Can you work these out from the model? Positions are in its coordinate system, mm. Face numbers are marked on the shaded views. A direction names the side the tool comes from. Coordinates: 2 decimals unless noted, no trailing zeros. Write each loop counter-clockwise with the first axis right and the second up, starting at its lowest first coordinate (ties: lowest second). Pieces come first, ordered by that corner, then holes. Notation, with made-up numbers: (-8.5, -34.75) -> (21.5, -34.75) arc R17 cw to (21.5, -18.75) -> close; hole circle Ø8 at (87, 71). An arc over 180 degrees is marked (long way). Answer as CSV lines item,"result". Start each with the question number.
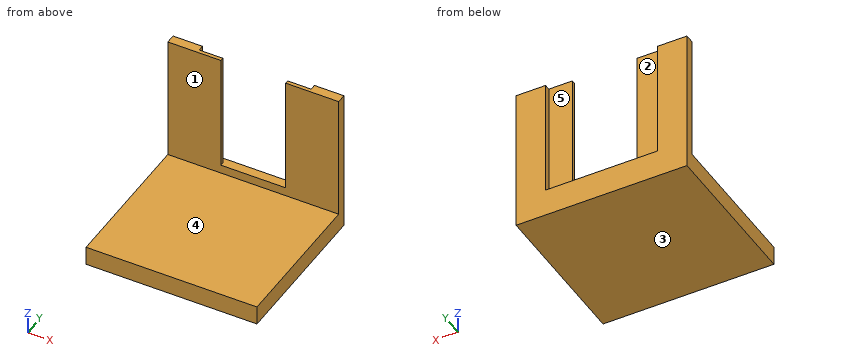
```python
from build123d import *

# Parameters (mm, degrees)
F0_W      = 38
F0_H      = 1.2
F1_DEPTH  = 20
F3_W      = 10
F3_H      = 20
F4_DEPTH  = 3.2
F5_W      = 10
F5_H      = 20
F6_DEPTH  = 3.2
F7_W      = 38
F7_H      = 2
F8_DEPTH  = 10
F2_W      = 22
F2_H      = 1.2
F9_DEPTH  = 20
F10_W     = 18
F10_H     = 7
F11_DEPTH = 50
F12_DEPTH = 20
F13_DEPTH = 40
F14_DEPTH = 0.5


with BuildPart() as f1:
    # F0 (on Top) → F1 (new body)
    with BuildSketch(Plane.XY):
        with Locations((19, 0.6)):
            Rectangle(F0_W, F0_H)
    extrude(amount=F1_DEPTH)

    # F3 (on face) → F4 (join)
    with BuildSketch(Plane.XZ):
        with Locations((-5, 10)):
            Rectangle(F3_W, F3_H)
    extrude(amount=-F4_DEPTH)

    # F5 (on face) → F6 (join)
    with BuildSketch(Plane.XZ):
        with Locations((43, 10)):
            Rectangle(F5_W, F5_H)
    extrude(amount=-F6_DEPTH)

    # F7 (on face) → F8 (join)
    with BuildSketch(Plane(origin=(0, 0, 0), x_dir=(1, 0, 0), z_dir=(0, 0, -1))):
        with Locations((19, -2.2)):
            Rectangle(F7_W, F7_H)
        Polygon((48, -3.2), (48, 0), (-10, 0), (-10, -3.2), (0, -3.2), (0, -1.2), (38, -1.2), (38, -3.2), align=None)
    extrude(amount=F8_DEPTH)

    # F2 (on face) → F9 (cut)
    with BuildSketch(Plane.XY.offset(20)):
        with Locations((19, 0.6)):
            Rectangle(F2_W, F2_H)
    extrude(amount=-F9_DEPTH, mode=Mode.SUBTRACT)

    # F10 (on face) → F11 (join)
    with BuildSketch(Plane.XZ):
        with Locations((-1, -6.5)):
            Rectangle(F10_W, F10_H)
    extrude(amount=F11_DEPTH)

    # F12 (add): faces of the model
    f12_faces = [f1.faces().sort_by_distance(p)[0] for p in [
        (40.9230769231, 1.3692307692, 20),
        (-2.9230769231, 1.3692307692, 20),
    ]]
    extrude(f12_faces, amount=F12_DEPTH)

    # F13 (add): a face of the model
    f13_faces = [f1.faces().sort_by_distance(p)[0] for p in [
        (8, -25, -6.5),
    ]]
    extrude(f13_faces, amount=F13_DEPTH)

    # F14 (cut): a face of the model
    f14_faces = [f1.faces().sort_by_distance(p)[0] for p in [
        (19, -23.4, -10),
    ]]
    extrude(f14_faces, amount=-F14_DEPTH, mode=Mode.SUBTRACT)


solid = f1.part
```
Q1. I need wall thicknesses on L1, parallel to Y at x = 2.5, z = 15; L2, parallel to Y at x = -2.5, z = 14; L3, parallel to Z at x = 22, y = -13.5. Which ranges of each line are inside material? Lowest first, please.
Q2. For pin 1 (21.5 mm diameter, centred on x = 30, z = 8.5, fed in from -Y); pin 2 (4 mm diameter, centred on x = 41, y = -15, fed in from +Z); pin 3 (2.5 mm diameter, centred on x = 16, y = 2.5, fed in from +Z), each with a flat end and sliding along its axis, tell me the tip position at first contact or that it passes through.
Q3. If we mould it in two halves opening along X, with no side actions, what happens to the marked faces 1 and 2? For each: released by +X, released by -X, zero draft, split by the parting line, or undercut.
Q4. Imagine slicing it at D-D (z = -1.5). Write out the boundary of the cut face in (x, y).
Q5. Imagine slicing it at B-B (x = 34.5). Write out the boundary of the cut face in (y, z).
Q6. Which directions (+Z, -Z, +X, -X, +Y, -Y) give clear straight access to the entire face, cutting with the end or side of a thin tool? Please do the marked faces 3, 4 and 5.
Q7. Imagine slicing it at A-A (z = 17). Write out the boundary of the cut face in (x, y).
Q8. Imagine slicing it at C-C (y = -5.5). Write out the boundary of the cut face in (x, z), then the cut area to 3 significant figures.
Entries:
1,L1,"0 to 1.2"
1,L2,"0 to 3.2"
1,L3,"-9.5 to -3"
2,pin 1,"y = 0"
2,pin 2,"z = -3"
2,pin 3,"z = 0"
3,face 1,"zero draft"
3,face 2,"undercut"
4,outline,"(-10, 0) -> (48, 0) -> (48, 3.2) -> (-10, 3.2) -> close"
5,outline,"(-50, -9.5) -> (3.2, -9.5) -> (3.2, 0) -> (1.2, 0) -> (1.2, 40) -> (0, 40) -> (0, -3) -> (-50, -3) -> close"
6,face 3,"-Z, +X, -X, +Y, -Y"
6,face 4,"+Z, +X, -X, -Y"
6,face 5,"+Z, +Y"
7,outline,"(-10, 0) -> (8, 0) -> (8, 1.2) -> (0, 1.2) -> (0, 3.2) -> (-10, 3.2) -> close; (30, 0) -> (48, 0) -> (48, 3.2) -> (38, 3.2) -> (38, 1.2) -> (30, 1.2) -> close"
8,outline,"(-10, -9.5) -> (48, -9.5) -> (48, -3) -> (-10, -3) -> close"
8,area,"377 mm2"
